The model under review builds one solid part; all positions refer to its coordinate system, in mm. Round coordinates to 2 decimals unless told otherwise and drop trailing zeros. Loops run counter-clockwise (first coordinate to the right, second up) from the corner with the lowest first, then second, coordinate; pieces in that order, holes last. Notation, with made-up numbers: (24.5, 20) -> (39.5, 20) arc R29 cw to (39.5, 55) -> close; hole circle Ø5 at (19.5, 57). An arc over 180 degrees is marked (long way). Return JSON: item names as keys, results as strings. Group by question number.
Autodesk Inventor part; units mm, degrees
ref_plane "YZ Plane" through (0, 0, 0) normal (1, 0, 0) x (0, 1, 0)
ref_plane "XZ Plane" through (0, 0, 0) normal (0, 1, 0) x (-1, 0, 0)
ref_plane "XY Plane" through (0, 0, 0) normal (0, 0, 1) x (1, 0, 0)
sketch "Sketch1" plane through (0, 0, 0) normal (0, 1, 0) x (-1, 0, 0)
  circle A0 centre (0, 0) radius 45
  dimension "d0" = 90
extrude "Extrusion1" add sketch "Sketch1" along normal blind 10
sketch "Sketch3" plane through (0, 10, 0) normal (0, 1, 0) x (1, 0, 0)
  circle A0 centre (0, 0) radius 50
  dimension "d5" = 100
extrude "Extrusion2" add sketch "Sketch3" along normal blind 5
sketch "Sketch4" plane through (0, 0, 0) normal (0, -1, 0) x (1, 0, 0)
  circle A0 centre (0, 0) radius 50
  dimension "d8" = 100
extrude "Extrusion3" add sketch "Sketch4" along normal blind 5
full round fillet "Full Round Fillet1" first side at (0, 0, -46.5023) centre faces at (-7.8142, 6.6667, -44.3163) second side at (0, 10, -46.5023)
sketch "Sketch5" plane through (0, 15, 0) normal (0, 1, 0) x (1, 0, 0)
  point P0 (0, 0)
  point P1 (0, 0)
hole "Hole1" at (0, 15, 0) at (0, 15, 0) direction (0, -1, 0) diameter 15 end through all
thread "Thread1"
properties part number "pump rotor"
1. Wall thickness on line 1 (Z direction, x = 0, y = 4.75); line 2 (Z direction, x = 0, y = 7.5); line 3 (Y direction, x = -31.5, z = -32.5): over which ranges is each line inside the solid? List them lowest first.
2. We need section C-C, the plane y = 8. Write out the cut boundary in (x, z), then the cut area to 3 significant figures.
3. For P1, Ø3, axis at y = 0.5, z = -7, coming from the -X side; P2, Ø17, axis at x = 0, z = 0, coming from the +Y side; P3, Ø3, axis at y = 12.5, z = -21.5, coming from the +X side; P4, Ø6, axis at x = -1, y = 1, coming from the -Z side, all flat-tipped, find the tip position at first contact; note any pin that passes through.
4. Draft analysis for pull direction X (two halves, no side actions). For faces 1 (the face through (-0.33, 4.86, -7.493)), 2 (the face through (-1, 15, 10)), 3 (the face through (47.69, 12.46, 15.02)), state which applies: pulls with the +X half, pulls with the -X half, needs draft (parallel to the pull), parting line crosses it, or undercut.
Check sheet entries:
{
 "1": {"line 1": "z = -45.01 to -7.5, 7.5 to 45.01", "line 2": "z = -45.67 to -7.5, 7.5 to 45.67", "line 3": "y = -5 to 3.41, 6.59 to 15"},
 "2": {"outline": "circle Ø92 at (0, 0); hole circle Ø15 at (0, 0)", "area": "6,470 mm²"},
 "3": {"P1": "stops at x = -49.69", "P2": "stops at y = 15", "P3": "stops at x = 45.83", "P4": "stops at z = -50"},
 "4": {"face 1": "undercut", "face 2": "needs draft", "face 3": "parting line crosses it"}
}
